from build123d import *

# Parameters (mm, degrees)
F0_W     = 0.8
F0_H     = 18
F0_R     = 80
F1_DEPTH = 2


with BuildPart() as f1:
    # F0 (on Top) → F1 (new body)
    with BuildSketch(Plane.XY):
        with BuildLine():
            Line((-96.8, 41), (-96.8, 59))
            ThreePointArc((-96.8, 59), (-98.8, 50), (-96.8, 41))
        make_face()
        with Locations((-96.4, -50)):
            Rectangle(F0_W, F0_H)
        with BuildLine():
            Line((96.8, 59), (96, 59))
            Line((96, 59), (96, 41))
            Line((96, 41), (96.8, 41))
            ThreePointArc((96.8, 41), (98.8, 50), (96.8, 59))
        make_face()
        with BuildLine():
            Line((-96.8, -59), (-96.8, -41))
            ThreePointArc((-96.8, -41), (-98.8, -50), (-96.8, -59))
        make_face()
        with BuildLine():
            ThreePointArc((96, 61), (85.748737, 85.748737), (61, 96))
            Line((61, 96), (47, 96))
            Line((47, 96), (47, 93))
            Line((47, 93), (40, 93))
            Line((40, 93), (40, 96))
            Line((40, 96), (-40, 96))
            Line((-40, 96), (-40, 93))
            Line((-40, 93), (-47, 93))
            Line((-47, 93), (-47, 96))
            Line((-47, 96), (-61, 96))
            ThreePointArc((-61, 96), (-85.748737, 85.748737), (-96, 61))
            Line((-96, 61), (-96, 59))
            Line((-96, 59), (-96, 41))
            Line((-96, 41), (-96, -41))
            Line((-96, -41), (-96, -59))
            Line((-96, -59), (-96, -61))
            ThreePointArc((-96, -61), (-85.748737, -85.748737), (-61, -96))
            Line((-61, -96), (-47, -96))
            Line((-47, -96), (-47, -93))
            Line((-47, -93), (-40, -93))
            Line((-40, -93), (-40, -96))
            Line((-40, -96), (40, -96))
            Line((40, -96), (40, -93))
            Line((40, -93), (47, -93))
            Line((47, -93), (47, -96))
            Line((47, -96), (61, -96))
            ThreePointArc((61, -96), (85.748737, -85.748737), (96, -61))
            Line((96, -61), (96, -59))
            Line((96, -59), (96, -41))
            Line((96, -41), (96, 41))
            Line((96, 41), (96, 59))
            Line((96, 59), (96, 61))
        make_face()
        Circle(F0_R, mode=Mode.SUBTRACT)
        with Locations((-96.4, 50)):
            Rectangle(F0_W, F0_H)
        with BuildLine():
            Line((96.8, -41), (96, -41))
            Line((96, -41), (96, -59))
            Line((96, -59), (96.8, -59))
            ThreePointArc((96.8, -59), (98.8, -50), (96.8, -41))
        make_face()
    extrude(amount=F1_DEPTH)


solid = f1.part
Geometry check sheet. Reference: the model listing, model coordinates, mm. Coordinates: 2 decimals unless noted, no trailing zeros. Order: outer loops, then holes, each group sorted by start corner. A loop starts at its lowest first (then second) coordinate and runs counter-clockwise, first axis right, second up. Notation, with made-up numbers: (49.25, 72.5) - (101.25, 72.5) arc R25 ccw to (101.25, 85.5) - close; hole circle Ø6 at (-18.75, 39). An arc over 180 degrees is marked (long way). One line per item, written item: value.
(1) Depth check by flat-ended pin: pin 1 Ø0.6 at (x, z) = (96.5, 1) entering from +Y; pin 2 Ø0.6 at (y, z) = (60, 0.5) entering from +X; pin 3 Ø1 at (y, z) = (-60.5, 0.5) entering from -X. Enter the tip coordinate at first touch or a pass-through.
Data:
pin 1: stops at y = 59
pin 2: stops at x = 96
pin 3: stops at x = -96
(2) Thickness scan on probe 1 along Y at (x, z) = (0, 0.5); probe 2 along X at (y, z) = (44, 1.1); probe 3 along X at (y, z) = (-74, 1.65). Record the ranges inside material, lowest first. Write a range as from..to.
Data:
probe 1: y = -96..-80, 80..96
probe 2: x = -97.94..-66.81, 66.81..97.94
probe 3: x = -93.5..-30.4, 30.4..93.5
(3) Sectioned sample at A-A (y = 0). Enter the section's corners in (x, z).
Data:
outline: (-96, 0) - (-80, 0) - (-80, 2) - (-96, 2) - close; (80, 0) - (96, 0) - (96, 2) - (80, 2) - close
(4) Release check for a two-part mould opening along X. For faces 1 (the face through (-67, 44, 2)), 2 (the face through (-17.34, -78.1, 0.99)), 3 (the face through (86.019, 85.475, 0.986)) record: +X half, -X half, draft (parallel to the pull), parting line (faces both ways), or undercut.
Data:
face 1: draft
face 2: undercut
face 3: +X half
